For this review, take the finished solid that the model builds, in its own axes (mm). Face numbers are marked on the shaded views. Round coordinates to 2 decimals unless told otherwise and drop trailing zeros. Write each loop counter-clockwise with the first axis right and the second up, starting at its lowest first coordinate (ties: lowest second). Pieces come first, ordered by that corner, then holes. Notation, with made-up numbers: (12.5, 0.5) -> (25.5, 0.5) arc R30 ccw to (25.5, 35.5) -> close; hole circle Ø4 at (66.5, 27). An arc over 180 degrees is marked (long way). Write each question's results on one line, items separated by ' | '. Start each with the question number.
Item 1: Clearance check with flat-ended pins moving along their axes: pin 1 (4.5 mm diameter, centred on y = -45.5, z = 21, fed in from +X); pin 2 (4.5 mm diameter, centred on y = -46, z = 33.5, fed in from -X); pin 3 (1.6 mm diameter, centred on x = 0.5, z = 23, fed in from -Y). State where each tip first meets the part, or that it passes through.
Item 2: Add section A-A (y = -43). State the section outline as (x, z) points.
Item 3: To check wall thickness, follow line 1 along X through (y, z) = (-44, 15); line 2 along Y through (x, z) = (0.25, 9); line 3 along Y through (x, z) = (2.5, 38). State the ranges of each line that lie inside material, in increasing order.
Item 4: The part is to be moulded in two halves that separate along X. For the marked faces 1 and 2, say which applies: +X half, -X half, draft (parallel to the pull), parting line (faces both ways), or undercut.
Item 5: Add section B-B (z = 20). State the section outline as (x, y) points (3 decimals).
Item 6: Add section D-D (x = 4.75). State the section outline as (y, z) points, plus the area to 3 significant figures.
Item 7: Add section C-C (y = -48). State the section outline as (x, z) points.
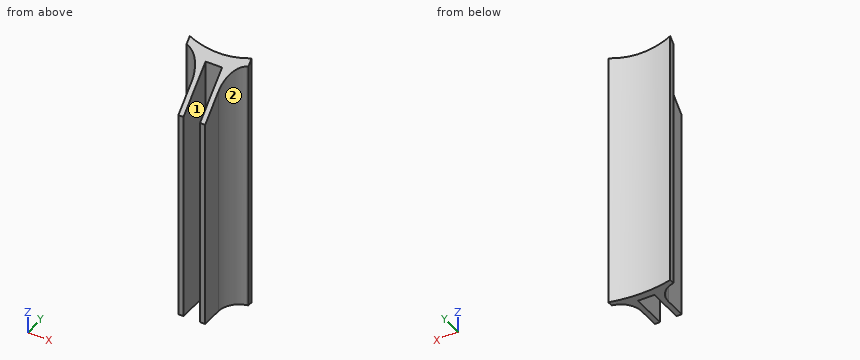
from build123d import *

# Parameters (mm, degrees)
PAD004_DEPTH            = 50
FILLET003_R             = 4
POCKET003_DEPTH         = 8.601
POCKET003_DEPTH_BACK    = 3.401
BODY005_PLACEMENT_ANGLE = 90


with BuildPart() as part:
    # Sketch008 → Pad004 (new body)
    with BuildSketch(Plane.XY):
        with BuildLine():
            ThreePointArc((24.269322, -6), (25, 0), (24.269322, 6))
            Line((24.269322, 6), (25.298221, 6))
            ThreePointArc((25.869673, 2.6), (25.640366, 4.309482), (25.298221, 6))
            Line((25.869673, 2.6), (33.451654, 2.6))
            Line((33.451654, 2.6), (33.451654, 1.6))
            Line((33.451654, 1.6), (26.451654, 1.6))
            Line((26.451654, 1.6), (26.451654, -1.6))
            Line((26.451654, -1.6), (33.451654, -1.6))
            Line((33.451654, -1.6), (33.451654, -2.6))
            Line((33.451654, -2.6), (25.869673, -2.6))
            ThreePointArc((25.298221, -6), (25.640366, -4.309482), (25.869673, -2.6))
            Line((24.269322, -6), (25.298221, -6))
        make_face()
    extrude(amount=PAD004_DEPTH)

    # Fillet003
    fillet003_edges = [part.edges().sort_by_distance(p)[0] for p in [
        (25.869673, -2.6, 25),
        (25.869673, 2.6, 25),
    ]]
    fillet(fillet003_edges, radius=FILLET003_R)

    # Sketch009 (on Face15 of Fillet003) → Pocket003 (cut, two sides)
    with BuildSketch(Plane.XZ.offset(2.6)) as pocket003_sk:
        Polygon((33.451654, 50), (33.451654, 40.817668), (24.269322, 50), align=None)
    extrude(amount=-POCKET003_DEPTH, mode=Mode.SUBTRACT)
    extrude(pocket003_sk.sketch, amount=POCKET003_DEPTH_BACK, mode=Mode.SUBTRACT)


with BuildPart() as part_1:
    # Body005 placement: moved
    add(part.part.moved(Location((0, -15, 0))).rotate(Axis((0, -15, 0), (0, 0, -1)), BODY005_PLACEMENT_ANGLE))


solid = part_1.part
Responses:
1) pin 1: stops at x = 2.73 | pin 2: stops at x = -2.63 | pin 3: stops at y = -41.45
2) outline: (-2.81, 0) -> (-1.6, 0) -> (-1.6, 46.27) -> (-2.81, 46.27) -> close; (1.6, 0) -> (2.81, 0) -> (2.81, 46.27) -> (1.6, 46.27) -> close
3) line 1: x = -2.61 to -1.6, 1.6 to 2.61 | line 2: y = -41.45 to -40 | line 3: y = -48.45 to -39.87
4) face 1: undercut | face 2: +X half
5) outline: (-6, -40.298) arc R26 ccw to (-5.72, -40.363) arc R4 cw to (-2.6, -44.265) -> (-2.6, -48.452) -> (-1.6, -48.452) -> (-1.6, -41.452) -> (1.6, -41.452) -> (1.6, -48.452) -> (2.6, -48.452) -> (2.6, -44.265) arc R4 cw to (5.72, -40.363) arc R26 ccw to (6, -40.298) -> (6, -39.269) arc R25 cw to (-6, -39.269) -> close
6) outline: (-40.72, 0) -> (-39.54, 0) -> (-39.54, 49.72) -> (-40.72, 48.55) -> close | area: 57.7 mm^2
7) outline: (-2.6, 0) -> (-1.6, 0) -> (-1.6, 41.27) -> (-2.6, 41.27) -> close; (1.6, 0) -> (2.6, 0) -> (2.6, 41.27) -> (1.6, 41.27) -> close
